The listing builds one solid part. Answer for the finished solid, in the listing's coordinates (mm). Round coordinates to 2 decimals unless told otherwise and drop trailing zeros. Loops run counter-clockwise (first coordinate to the right, second up) from the corner with the lowest first, then second, coordinate; pieces in that order, holes last. Notation, with made-up numbers: M 64,32 L 93,32 A14 ccw 93,44 Z; hole C -29.75,-11 d11. An arc over 180 degrees is marked long. Put each result on its own line as item: value. Start each with the question number.
(1) Straight lines are drawn through the part: line 1 (X direction, y = 27, z = -19.5); line 2 (Z direction, x = 92, y = 8.5); line 3 (Z direction, x = -225.5, y = -17.5). For each, find the intervals that lie inside material, in ascending order.
(2) Section B-B, the plane z = -196.5 is taken. Determine the outline of the cut face in (x, y).
(3) Section A-A, the plane x = 9 is taken. Determine the outline of the cut face in (y, z), then the cut area to 3 significant figures.
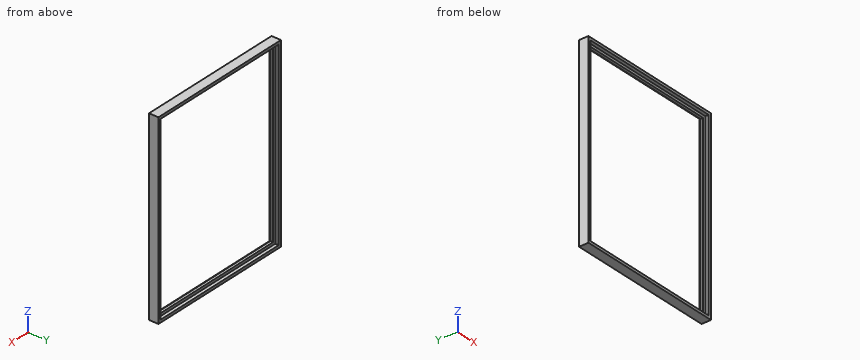
Autodesk Inventor part; units mm, degrees
ref_plane "YZ Plane" through (0, 0, 0) normal (1, 0, 0) x (0, 1, 0)
ref_plane "XZ Plane" through (0, 0, 0) normal (0, 1, 0) x (-1, 0, 0)
ref_plane "XY Plane" through (0, 0, 0) normal (0, 0, 1) x (1, 0, 0)
sketch "Sketch1" plane through (0, 0, 0) normal (0, 1, 0) x (-1, 0, 0)
  line L0 (533, 674) -> (-533, 674)
  line L1 (-533, 674) -> (-533, -674)
  line L2 (-533, -674) -> (533, -674)
  line L3 (533, -674) -> (533, 674)
  line L4 (533, 674) -> (-533, -674) construction
  line L5 (-533, 674) -> (533, -674) construction
  line L6 (553, 694) -> (-553, 694)
  line L7 (-553, 694) -> (-553, -694)
  line L8 (-553, -694) -> (553, -694)
  line L9 (553, -694) -> (553, 694)
  line L10 (553, 694) -> (-553, -694) construction
  line L11 (-553, 694) -> (553, -694) construction
  line L12 (513, 654) -> (-513, 654)
  line L13 (-513, 654) -> (-513, -654)
  line L14 (-513, -654) -> (513, -654)
  line L15 (513, -654) -> (513, 654)
  line L16 (513, 654) -> (-513, -654) construction
  line L17 (-513, 654) -> (513, -654) construction
  point P0 (0, 0)
  dimension "d0" = 1066
  dimension "d1" = 1348
  dimension "d2" = 1106
  dimension "d3" = 1388
  dimension "d4" = 1026
  dimension "d5" = 1308
extrude "Extrusion2" add sketch "Sketch1" along normal mid plane 20 contours L3 L2 L1 L0
extrude "Extrusion3" add sketch "Sketch1" along normal mid plane 70 contours L9 L8 L7 L6
properties part number "solar panels holder"
Recorded:
1. line 1: x = -553 to -533, 533 to 553
1. line 2: z = -694 to -654, 654 to 694
1. line 3: z = -694 to -674, 674 to 694
2. outline: M -553,-35 L -533,-35 L -533,-10 L -513,-10 L -513,10 L -533,10 L -533,35 L -553,35 Z; M 513,-10 L 533,-10 L 533,-35 L 553,-35 L 553,35 L 533,35 L 533,10 L 513,10 Z
3. outline: M -35,-694 L 35,-694 L 35,-674 L 10,-674 L 10,-654 L -10,-654 L -10,-674 L -35,-674 Z; M -35,674 L -10,674 L -10,654 L 10,654 L 10,674 L 35,674 L 35,694 L -35,694 Z
3. area: 3,600 mm²
